Check sheet for the drawn part. Datum: minimum x, y, z corner. Units: mm. A direction names the side the tool comes from. Coordinates: 2 decimals unless noted, no trailing zeros. Write each loop counter-clockwise with the first axis right and the second up, starting at its lowest first coordinate (ties: lowest second). Pieces come first, ordered by that corner, then holes. Notation, with made-up numbers: (27, 37.5) - (47, 37.5) arc R24 cw to (47, 76.5) - close; hole circle Ø3 at (29, 83). An arc over 180 degrees is marked (long way). Use one line per item in the form item = value. Start each with the question number.
1. Cross-section at D-D on z = 5.25. Record the boundary of the cut face in (x, y), then the cut area to 3 significant figures.
2. Cross-section at C-C on z = 8. Record the boundary of the cut face in (x, y), then the cut area to 3 significant figures.
3. Cross-section at A-A on y = 0.75. Record the boundary of the cut face in (x, z), then the cut area to 4 significant figures.
4. Scan lines: line 1 along X through (y, z) = (0.7, 3.5); line 2 along Y through (x, z) = (0.7, 8). Record each from-to range of solid material in increasing order.
5. Tool access check on the marked faces 1, 2 and 3. Record the directions out of +Z, -Z, +X, -X, +Y, -Y that give a thin tool (end or side, any length) a straight path to the whole face; none if there is none.
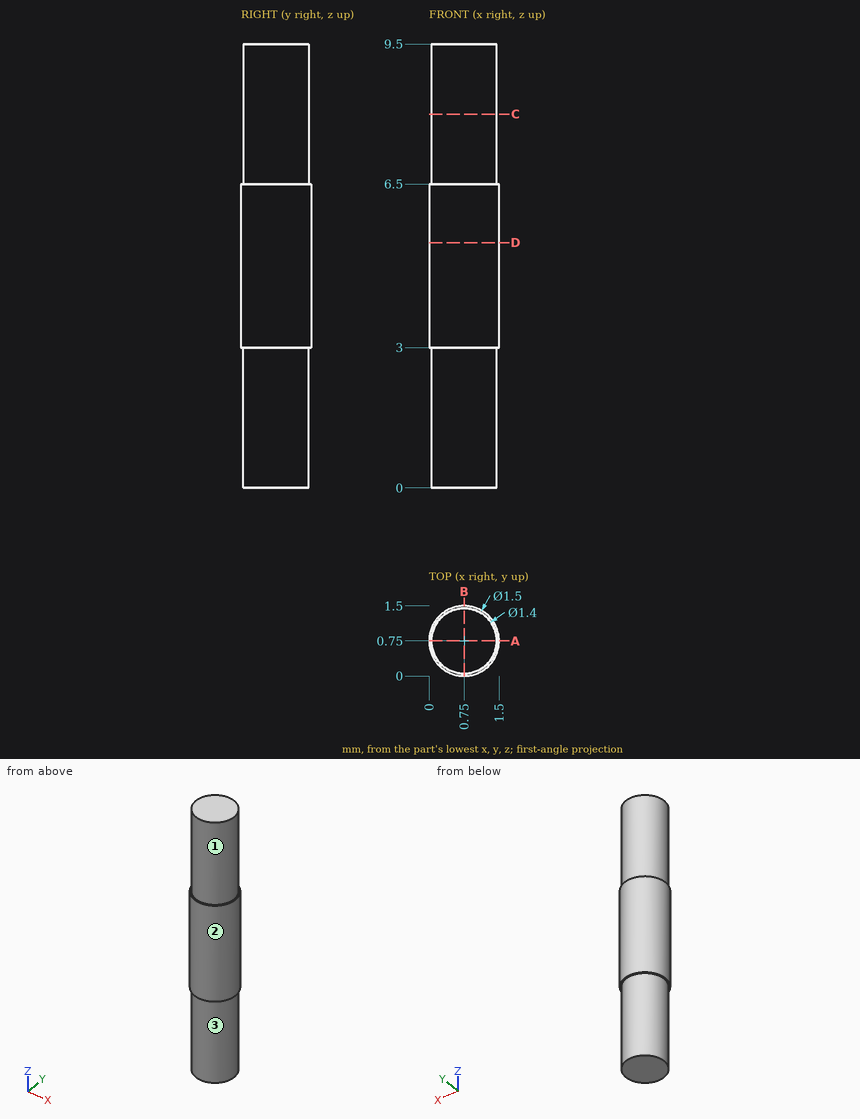
Final values:
q1.outline = circle Ø1.5 at (0.75, 0.75)
q1.area = 1.77 mm²
q2.outline = circle Ø1.4 at (0.75, 0.75)
q2.area = 1.54 mm²
q3.outline = (0, 3) - (0.05, 3) - (0.05, 0) - (1.45, 0) - (1.45, 3) - (1.5, 3) - (1.5, 6.5) - (1.45, 6.5) - (1.45, 9.5) - (0.05, 9.5) - (0.05, 6.5) - (0, 6.5) - close
q3.area = 13.65 mm²
q4.line_1 = 0 to 1.5
q4.line_2 = 0.05 to 1.45
q5.face_1 = +Z
q5.face_2 = +Z, -Z
q5.face_3 = -Z
